Source: three-view drawing plus pictorial views. Frame: mm from the lowest corner of the part. Give positions to 0.01 mm unless a question says otherwise; leave off trailing zeros. Loops run counter-clockwise (first coordinate to the right, second up) from the corner with the lowest first, then second, coordinate; pieces in that order, holes last. Notation, with made-up numbers: (45, 39.5) -> (76, 39.5) arc R21 cw to (76, 71.5) -> close; hole circle Ø8 at (16, 26.5). An arc over 180 degrees is marked (long way). One line per item, written item: value. Start each with the question number.
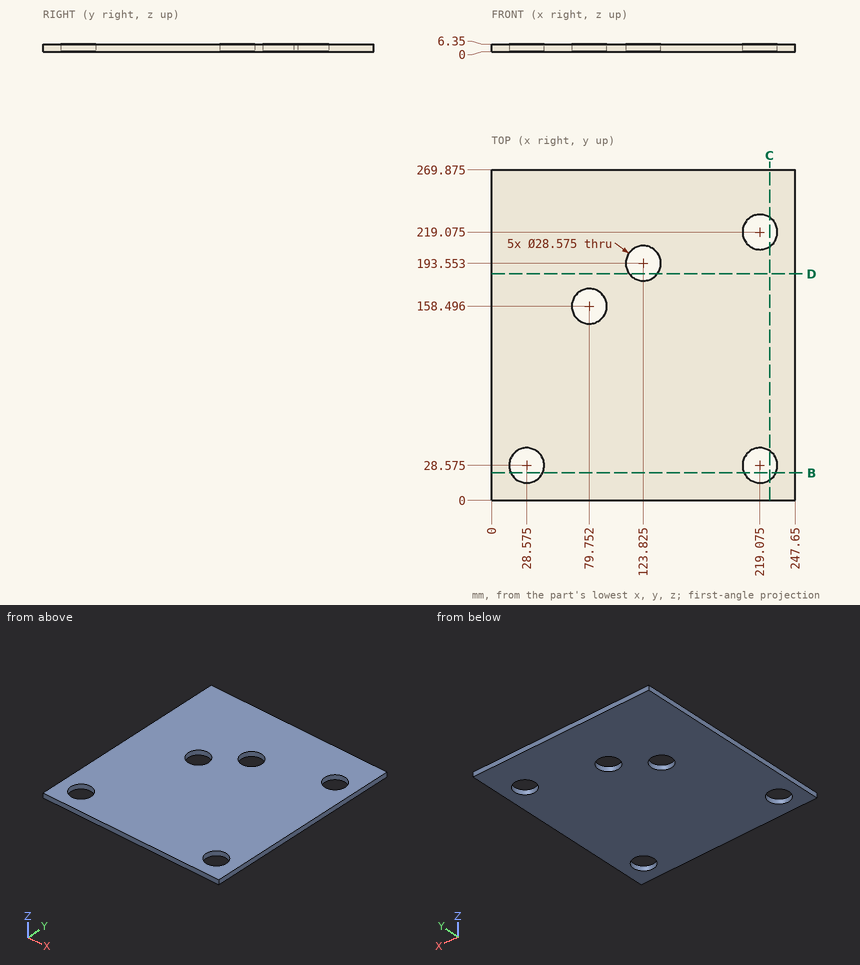
Item 1: Section C-C, the plane x = 227. State how many separate pieces and enclosed holes the cut face has, then the cut area to 3 significant figures.
Item 2: Pin query (flat end, axial travel): pin 1 (3 mm diameter, centred on x = 118, y = 142, fed in from -Z). Return the tip coordinate at first contact, or that it passes through.
Item 3: Section B-B, the plane y = 22.5. Output: boundary loops of the cut face in (x, z).
Item 4: Ray query, line 1 along X through (y, z) = (191, 5.25); line 2 along X through (y, z) = (158, 6); line 3 along Y through (x, z) = (41, 5.5) (1 decimal). Return the intervals inside material, ascending. Write a range as [from, to].
Item 5: Section D-D, the plane y = 185. Output: boundary loops of the cut face in (x, z), then the cut area to 3 significant figures.
Geometry check:
1. separate pieces: 3
1. enclosed holes: 0
1. area: 1,410 mm2
2. pin 1: stops at z = 0
3. outline: (0, 0) -> (15.64, 0) -> (15.64, 6.35) -> (0, 6.35) -> close; (41.51, 0) -> (206.14, 0) -> (206.14, 6.35) -> (41.51, 6.35) -> close; (232.01, 0) -> (247.65, 0) -> (247.65, 6.35) -> (232.01, 6.35) -> close
4. line 1: x = [0, 109.77], [137.88, 247.65]
4. line 2: x = [0, 65.47], [94.03, 247.65]
4. line 3: y = [0, 21.5], [35.6, 269.9]
5. outline: (0, 0) -> (112.38, 0) -> (112.38, 6.35) -> (0, 6.35) -> close; (135.27, 0) -> (247.65, 0) -> (247.65, 6.35) -> (135.27, 6.35) -> close
5. area: 1,430 mm2
